Autodesk Inventor part; units mm, degrees
ref_plane "YZ Plane" through (0, 0, 0) normal (1, 0, 0) x (0, 1, 0)
ref_plane "XZ Plane" through (0, 0, 0) normal (0, 1, 0) x (-1, 0, 0)
ref_plane "XY Plane" through (0, 0, 0) normal (0, 0, 1) x (1, 0, 0)
sketch "Sketch1" plane through (0, 0, 0) normal (0, 1, 0) x (-1, 0, 0)
  line L0 (0, -14.0533) -> (0, 14.0533) construction
  line L1 (4.9803, 0) -> (-4.9803, 0) construction
  line L2 (25, 25) -> (-25, 25)
  line L3 (-25, 25) -> (-25, -25)
  line L4 (-25, -25) -> (25, -25)
  line L5 (25, -25) -> (25, 25)
  arc A0 (7.0711, 2.5) -> (7.0711, -2.5) centre (0, 0) ccw
  line L6 (9.8, 2.5) -> (7.0711, 2.5)
  line L7 (7.0711, -2.5) -> (9.8, -2.5)
  line L8 (9.8, -2.5) -> (9.8, 2.5)
  dimension "d0" = 50
  dimension "d1" = 15
  dimension "d18" = 5
  dimension "d19" = 9.8
extrude "Extrusion1" add sketch "Sketch1" along normal blind 4
sketch "Sketch2" plane through (0, 4, 0) normal (0, 1, 0) x (1, 0, 0)
  line L0 (25, 25) -> (-25, 25)
  line L1 (-25, 25) -> (-25, -25)
  line L2 (-25, -25) -> (25, -25)
  line L3 (25, -25) -> (25, 25)
  point P0 (0, 0)
  point P1 (-15, -15)
  point P2 (-15, 15)
  point P3 (15, 15)
  point P4 (15, -15)
  dimension "d4" = 10
  dimension "d5" = 10
  dimension "d6" = 10
  dimension "d7" = 10
hole "Hole1" at (-15, 4, 15) at (-15, 4, -15) at (15, 4, -15) at (15, 4, 15) direction (0, -1, 0) diameter 6.6 end through all
chamfer "Chamfer1" distance 1 angle 45 8 edges at (-25, 2, 25) (25, 2, 25) (25, 2, -25) (0, 4, -25) (-25, 4, 0) (0, 4, 25) (25, 4, 0) (-25, 2, -25)
properties part number "FlanschV1"
Read the model definition and answer for the solid it produces. Units are mm, in the model's axes. A direction names the side the tool comes from. Give positions to 0.01 mm unless a question says otherwise; leave off trailing zeros. Write each loop counter-clockwise with the first axis right and the second up, starting at its lowest first coordinate (ties: lowest second). Pieces come first, ordered by that corner, then holes. Notation, with made-up numbers: (-15, 53.25) - (-8, 53.25) arc R17 ccw to (-8, 74.25) - close; hole circle Ø4 at (67, 82.25). An arc over 180 degrees is marked (long way). Use CSV: the item, a comma, the result in double quotes. Start each with the question number.
Item 1: The part is cut by section A-A, the plane z = 0. Give the vertices of the cut face in (x, y), and give its area (3 significant figures).
Item 2: The mould has two halves that part along Z. Classify faces 1 (the flat face through (0, 1, 25)), 2 (the flat face through (0, 1, -25)), 3 (the flat face through (-8, 2, -2.5)): pulls with the +Z half, pulls with the -Z half, needs draft (parallel to the pull), parting line crosses it, or undercut.
Item 3: The part is cut by section B-B, the plane x = -8. Give the vertices of the cut face in (y, z).
Item 4: The part is cut by section D-D, the plane z = 15. Give the vertices of the cut face in (x, y), and give its area (3 significant figures).
Item 5: For faces 4 (the flat face through (-8, 2, 2.5)), 5 (the flat face through (-25, 1, 0)), determine the directions among +Z, -Z, +X, -X, +Y, -Y from which every point of the face is accessible in a straight line to the end or side of a thin tool.
Item 6: Consider line 1 (Z direction, x = -15, y = 1.45); line 2 (Z direction, x = -17, y = 3.05). Determine where each line is inside the solid, lowest interval first.
Item 7: The part is cut by section C-C, the plane x = -15. Give the vertices of the cut face in (y, z).
Taken from the geometry:
1,outline,"(-25, 0) - (-9.8, 0) - (-9.8, 4) - (-24, 4) - (-25, 3) - close; (7.5, 0) - (25, 0) - (25, 3) - (24, 4) - (7.5, 4) - close"
1,area,"130 mm2"
2,face 1,"pulls with the +Z half"
2,face 2,"pulls with the -Z half"
2,face 3,"undercut"
3,outline,"(0, -25) - (3, -25) - (4, -24) - (4, -2.5) - (0, -2.5) - close; (0, 2.5) - (4, 2.5) - (4, 24) - (3, 25) - (0, 25) - close"
4,outline,"(-25, 0) - (-18.3, 0) - (-18.3, 4) - (-24, 4) - (-25, 3) - close; (-11.7, 0) - (11.7, 0) - (11.7, 4) - (-11.7, 4) - close; (18.3, 0) - (25, 0) - (25, 3) - (24, 4) - (18.3, 4) - close"
4,area,"146 mm2"
5,face 4,"+Y, -Y"
5,face 5,"+Z, -Z, -X, +Y, -Y"
6,line 1,"-25 to -18.3, -11.7 to 11.7, 18.3 to 25"
6,line 2,"-24.95 to -17.62, -12.38 to 12.38, 17.62 to 24.95"
7,outline,"(0, -25) - (3, -25) - (4, -24) - (4, -18.3) - (0, -18.3) - close; (0, -11.7) - (4, -11.7) - (4, 11.7) - (0, 11.7) - close; (0, 18.3) - (4, 18.3) - (4, 24) - (3, 25) - (0, 25) - close"
